Geometry check sheet. Reference: the model listing, model coordinates, mm. Face numbers are marked on the shaded views. Coordinates: 2 decimals unless noted, no trailing zeros. Write each loop counter-clockwise with the first axis right and the second up, starting at its lowest first coordinate (ties: lowest second). Pieces come first, ordered by that corner, then holes. Notation, with made-up numbers: (49, -12.75) -> (96, -12.75) arc R22 ccw to (96, 13.25) -> close; hole circle Ø9 at (36, 35.5). An arc over 180 degrees is marked (long way). Answer in a Markdown table with one row per item. Add a question column.
1. Scan lines: L1, parallel to Z at x = -0.75, y = 0; L2, parallel to Y at x = -0.25, z = 25.4; L3, parallel to Y at x = -1.25, z = 25.4. Record each from-to range of solid material in increasing order. Write a range as from..to.
2. Cross-section at C-C on z = 26. Record the cut outline in (x, y), and give its area (3 significant figures).
3. Mould release check, pull along Z, two halves, no side actions. Record for the marked faces 1, 2 and 3: pulls with the +Z half, pulls with the -Z half, needs draft (parallel to the pull), parting line crosses it, or undercut.
4. Depth check by flat-ended pin: P1, Ø4, axis at x = 4.5, z = 10.5, coming from the +Y side; P2, Ø1, axis at y = -2, z = 29.5, coming from the +X side; P3, Ø1, axis at x = -3, z = 34, coming from the -Y side. Enter the tip coordinate at first touch or a pass-through.
5. Cross-section at D-D on y = -4. Record the cut outline in (x, z), and give its area (3 significant figures).
6. Cross-section at B-B on x = -4.5. Record the cut outline in (y, z).
7. Cross-section at A-A on y = 0. Record the cut outline in (x, z), and give its area (3 significant figures).
```python
from build123d import *

# Parameters (mm, degrees)
F0_R      = 6.35
F1_DEPTH  = 50.8
F2_R      = 1.651
F3_DEPTH  = 6.351
F3_FACE_R = 1.651
F4_DEPTH  = 25.4


with BuildPart() as f1:
    # F0 (on Top) → F1 (new body)
    with BuildSketch(Plane.XY):
        Circle(F0_R)
    extrude(amount=F1_DEPTH)

    # F2 (on Right) → F3 (cut, through all)
    with BuildSketch(Plane.YZ):
        with Locations((0, 25.4)):
            Circle(F2_R)
    extrude(amount=-F3_DEPTH, mode=Mode.SUBTRACT)

    # F3_face (on face) → F4 (cut)
    with BuildSketch(Plane(origin=(0, 0, 25.4), x_dir=(0, 1, 0), z_dir=(-1, 0, 0))):
        Circle(F3_FACE_R)
    extrude(amount=-F4_DEPTH, mode=Mode.SUBTRACT)


solid = f1.part
```
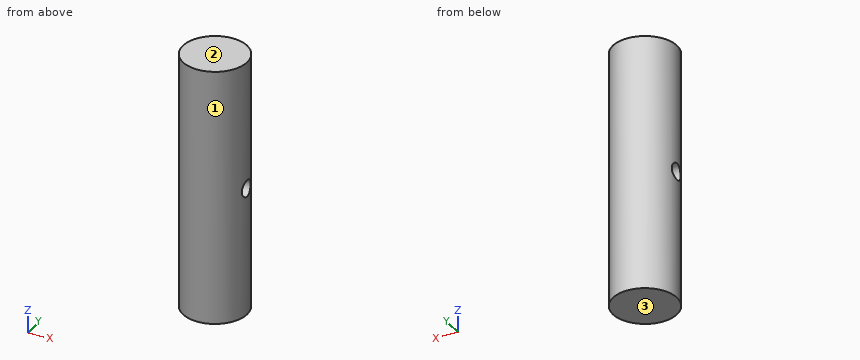
Results found:
| question | item | result |
|---|---|---|
| 1 | L1 | z = 0..23.75, 27.05..50.8 |
| 1 | L2 | y = -6.35..-1.65, 1.65..6.35 |
| 1 | L3 | y = -6.23..-1.65, 1.65..6.23 |
| 2 | outline | (-6.16, -1.54) arc R6.35 ccw to (6.16, -1.54) -> close; (-6.16, 1.54) -> (6.16, 1.54) arc R6.35 ccw to start |
| 2 | area | 88.0 mm^2 |
| 3 | face 1 | needs draft |
| 3 | face 2 | pulls with the +Z half |
| 3 | face 3 | pulls with the -Z half |
| 4 | P1 | stops at y = 5.84 |
| 4 | P2 | stops at x = 6.17 |
| 4 | P3 | stops at y = -5.84 |
| 5 | outline | (-4.93, 0) -> (4.93, 0) -> (4.93, 50.8) -> (-4.93, 50.8) -> close |
| 5 | area | 501 mm^2 |
| 6 | outline | (-4.48, 0) -> (4.48, 0) -> (4.48, 50.8) -> (-4.48, 50.8) -> close; hole circle Ø3.3 at (0, 25.4) |
| 7 | outline | (-6.35, 0) -> (6.35, 0) -> (6.35, 23.75) -> (-6.35, 23.75) -> close; (-6.35, 27.05) -> (6.35, 27.05) -> (6.35, 50.8) -> (-6.35, 50.8) -> close |
| 7 | area | 603 mm^2 |
